For this review, take the finished solid that the model builds, in its own axes (mm). A direction names the side the tool comes from. Round coordinates to 2 decimals unless told otherwise and drop trailing zeros. Order: outer loops, then holes, each group sorted by start corner. A loop starts at its lowest first (then second) coordinate and runs counter-clockwise, first axis right, second up. Notation, with made-up numbers: M 32.25,50 L 71.25,50 A25 cw 71.25,64 Z; hole C 57,25 d6. An arc over 180 degrees is marked long. Use a Markdown table: item, result.
from build123d import *

# Parameters (mm, degrees)
F1_R     = 7.5
F2_DEPTH = 5


with BuildPart() as f2:
    # F1 (on Top) → F2 (new body)
    with BuildSketch(Plane.XY):
        Polygon((80.296967, 71.212121), (75.296967, 71.212121), (50.296967, 71.212121), (50.296967, 51.212121), (45.296967, 51.212121), (45.296967, 71.212121), (40.296967, 71.212121), (40.296967, 61.212121), (-20.703033, 61.212121), (-20.703033, 56.212121), (-27.703033, 56.212121), (-27.703033, 61.212121), (-34.703033, 61.212121), (-34.703033, 41.212121), (-27.703033, 41.212121), (-27.703033, 46.212121), (-20.703033, 46.212121), (-20.703033, 41.212121), (40.296967, 41.212121), (40.296967, 31.212121), (85.296967, 31.212121), (85.296967, 71.212121), align=None)
        with Locations((63.296967, 51.212121)):
            Circle(F1_R, mode=Mode.SUBTRACT)
    extrude(amount=F2_DEPTH)


solid = f2.part
Q1. Clearance check with flat-ended pins moving along their axes: pin 1 (2 mm diameter, centred on x = 38, z = 3.5, fed in from +Y); pin 2 (2.5 mm diameter, centred on x = -30, z = 1.5, fed in from -Y); pin 3 (2.5 mm diameter, centred on y = 64.5, z = 3, fed in from -X). State where each tip first meets the part, or that it passes through.
Determined:
| item | result |
|---|---|
| pin 1 | stops at y = 61.21 |
| pin 2 | stops at y = 41.21 |
| pin 3 | stops at x = 40.3 |
Q2. Machinability: for faces 1 (the flat face through (-27.703, 59, 2)), 2 (the flat face through (-31, 61.212, 2)), 3 (the flat face through (-20.703, 44, 2)), 4 (the flat face through (9, 41.212, 2)), 5 (the flat face through (24, 51, 0)), which of the approach directions +Z, -Z, +X, -X, +Y, -Y give a long, thin tool a straight path to every point of the face, cutting with its end or side? Answer none if there is none.
Determined:
| item | result |
|---|---|
| face 1 | +Z, -Z, +Y |
| face 2 | +Z, -Z, -X, +Y |
| face 3 | +Z, -Z, -Y |
| face 4 | +Z, -Z, -X, -Y |
| face 5 | -Z, +X, -X, +Y, -Y |
Q3. Add section B-B (y = 35.5). Write out the cut boundary in (x, z), then the cut area to 3 significant figures.
Determined:
| item | result |
|---|---|
| outline | M 40.3,0 L 85.3,0 L 85.3,5 L 40.3,5 Z |
| area | 225 mm^2 |
Q4. Add section A-A (z = 3.75). Write out the cut boundary in (x, y).
Determined:
| item | result |
|---|---|
| outline | M -34.7,41.21 L -27.7,41.21 L -27.7,46.21 L -20.7,46.21 L -20.7,41.21 L 40.3,41.21 L 40.3,31.21 L 85.3,31.21 L 85.3,71.21 L 50.3,71.21 L 50.3,51.21 L 45.3,51.21 L 45.3,71.21 L 40.3,71.21 L 40.3,61.21 L -20.7,61.21 L -20.7,56.21 L -27.7,56.21 L -27.7,61.21 L -34.7,61.21 Z; hole C 63.3,51.21 d15 |
Q5. Wall thickness on line 1 along X through (y, z) = (60, 3.5); line 2 along Y through (x, z) = (63, 1.9); line 3 along X through (y, z) = (67.5, 1.45): over which ranges is each line inside the solid? List them lowest first. Write a range as [from, to].
Determined:
| item | result |
|---|---|
| line 1 | x = [-34.7, -27.7], [-20.7, 45.3], [50.3, 85.3] |
| line 2 | y = [31.21, 43.72], [58.71, 71.21] |
| line 3 | x = [40.3, 45.3], [50.3, 85.3] |
Q6. Draft analysis for pull direction Y (two halves, no side actions). For faces 6 (the flat face through (43, 71.212, 2)), 7 (the cylindrical face through (70.225, 48.34, 2.465)), 8 (the flat face through (-31, 41.212, 2)), 9 (the flat face through (-27.703, 44, 2)), state which applies: pulls with the +Y half, pulls with the -Y half, needs draft (parallel to the pull), parting line crosses it, or undercut.
Determined:
| item | result |
|---|---|
| face 6 | pulls with the +Y half |
| face 7 | undercut |
| face 8 | pulls with the -Y half |
| face 9 | needs draft |
Q7. Add section C-C (x = -13). Write out the cut boundary in (y, z).
Determined:
| item | result |
|---|---|
| outline | M 41.21,0 L 61.21,0 L 61.21,5 L 41.21,5 Z |
